from build123d import *

# Parameters (mm, degrees)
F0_W     = 20
F0_H     = 20
F1_DEPTH = 40
F2_R     = 4.5
F3_DEPTH = 7
F4_R     = 4.5
F5_DEPTH = 7
F6_R     = 1


with BuildPart() as f1:
    # F0 (on Front) → F1 (new body)
    with BuildSketch(Plane.XZ):
        Rectangle(F0_W, F0_H)
    extrude(amount=F1_DEPTH)

    # F2 (on face) → F3 (join)
    with BuildSketch(Plane(origin=(0, 0, 0), x_dir=(-1, 0, 0), z_dir=(0, 1, 0))):
        Circle(F2_R)
    extrude(amount=F3_DEPTH)

    # F4 (on face) → F5 (join)
    with BuildSketch(Plane.XZ.offset(40)):
        Circle(F4_R)
    extrude(amount=F5_DEPTH)

    # F6
    f6_edges = [f1.edges().sort_by_distance(p)[0] for p in [
        (-4.5, -47, 0),
        (4.5, 7, 0),
    ]]
    fillet(f6_edges, radius=F6_R)


solid = f1.part
Here's how the part is built. I have some questions about the finished solid (model axes, mm). A direction names the side the tool comes from. Round coordinates to 2 decimals unless told otherwise and drop trailing zeros. Loops run counter-clockwise (first coordinate to the right, second up) from the corner with the lowest first, then second, coordinate; pieces in that order, holes last.
1. If we section it at D-D on x = -5.5: Write out the boundary of the cut face in (y, z), plus the area to 3 significant figures.
Answer list:
outline: (-40, -10) - (0, -10) - (0, 10) - (-40, 10) - close
area: 800 mm2
2. If we section it at C-C on z = -6: Write out the boundary of the cut face in (x, y), plus the area to 3 significant figures.
Answer list:
outline: (-10, -40) - (10, -40) - (10, 0) - (-10, 0) - close
area: 800 mm2
3. If we section it at A-A on z = 0: Write out the boundary of the cut face in (x, y).
Answer list:
outline: (-10, -40) - (-4.5, -40) - (-4.5, -46) arc R1 ccw to (-3.5, -47) - (3.5, -47) arc R1 ccw to (4.5, -46) - (4.5, -40) - (10, -40) - (10, 0) - (4.5, 0) - (4.5, 6) arc R1 ccw to (3.5, 7) - (-3.5, 7) arc R1 ccw to (-4.5, 6) - (-4.5, 0) - (-10, 0) - close
4. If we section it at B-B on x = 0: Write out the boundary of the cut face in (y, z), plus the area to 3 significant figures.
Answer list:
outline: (-47, -3.5) arc R1 ccw to (-46, -4.5) - (-40, -4.5) - (-40, -10) - (0, -10) - (0, -4.5) - (6, -4.5) arc R1 ccw to (7, -3.5) - (7, 3.5) arc R1 ccw to (6, 4.5) - (0, 4.5) - (0, 10) - (-40, 10) - (-40, 4.5) - (-46, 4.5) arc R1 ccw to (-47, 3.5) - close
area: 925 mm2
5. For P1, Ø1.5, axis at x = -3.5, z = -1, coming from the -Y side; P2, Ø5, axis at x = 6.5, z = -3, coming from the +Y side; P3, Ø3, axis at x = -6, z = 6.5, coming from the -Y side, each with a flat end and sliding along its axis, tell me the tip position at first contact or that it passes through.
Answer list:
P1: stops at y = -47
P2: stops at y = 0
P3: stops at y = -40
6. If I drill on line 1 along Y through (x, z) = (5.25, 3); line 2 along X through (y, z) = (3.5, 3.75); line 3 along X through (y, z) = (4, 1.75), over which ranges is the centre line in solid material (lowest first)?
Answer list:
line 1: y = -40 to 0
line 2: x = -2.49 to 2.49
line 3: x = -4.15 to 4.15
7. Which directions (+Z, -Z, +X, -X, +Y, -Y) give clear straight access to the entire face, cutting with the end or side of a thin tool? Please do faces 1 (the face through (0, -20, -10)), 2 (the face through (0.59, 2.96, 4.46)), 3 (the face through (0, -40, 5)).
Answer list:
face 1: -Z, +X, -X, +Y, -Y
face 2: +Y
face 3: -Y
